from build123d import *

# Parameters (mm, degrees)
SKETCH1_W           = 10
SKETCH1_H           = 10
BOSS_EXTRUDE1_DEPTH = 8
SKETCH2_W           = 4
SKETCH2_H           = 3
CUT_EXTRUDE1_DEPTH  = 11
SKETCH3_W           = 1.504859188
SKETCH3_H           = 7
BOSS_EXTRUDE2_DEPTH = 3.5
FILLET1_R           = 2


with BuildPart() as part:
    # Sketch1 → Boss-Extrude1 (new body)
    with BuildSketch(Plane.XY):
        Rectangle(SKETCH1_W, SKETCH1_H)
    extrude(amount=BOSS_EXTRUDE1_DEPTH)

    # Sketch2 → Cut-Extrude1 (cut, through all)
    with BuildSketch(Plane.XZ.offset(5)):
        with Locations((0, 4)):
            Rectangle(SKETCH2_W, SKETCH2_H)
    extrude(amount=-CUT_EXTRUDE1_DEPTH, mode=Mode.SUBTRACT)

    # Sketch3 → Boss-Extrude2 (add)
    with BuildSketch(Plane.XY.offset(8)):
        Rectangle(SKETCH3_W, SKETCH3_H)
    extrude(amount=BOSS_EXTRUDE2_DEPTH)

    # Fillet1
    fillet1_edges = [part.edges().sort_by_distance(p)[0] for p in [
        (0, -5, 0),
        (-5, 0, 0),
        (0, 5, 0),
        (5, 0, 0),
        (5, -5, 4),
        (-5, -5, 4),
        (-5, 5, 4),
        (5, 5, 4),
    ]]
    fillet(fillet1_edges, radius=FILLET1_R)


solid = part.part
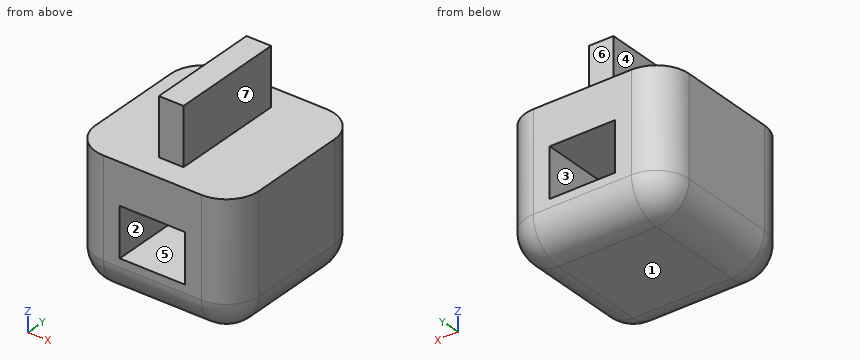
Can you work these out from the model? Positions are in its coordinate system, mm. Face numbers are marked on the shaded views. A direction names the side the tool comes from. Round coordinates to 2 decimals unless told otherwise and drop trailing zeros. Write each loop counter-clockwise with the first axis right and the second up, starting at its lowest first coordinate (ties: lowest second). Pieces come first, ordered by that corner, then holes. Notation, with made-up numbers: M 36,-34.5 L 57,-34.5 A8 cw 57,-22.5 Z; hole C 37,84.25 d4. An arc over 180 degrees is marked long. Use CSV: the item, a comma, the result in double quotes.
(1) We'd pull the mould along Z, two halves only. Please class the marked faces 1, 2, 3 and 4: +Z half, -Z half, draft (parallel to the pull), parting line (faces both ways), or undercut.
Check values:
face 1,"-Z half"
face 2,"undercut"
face 3,"undercut"
face 4,"draft"
(2) Imagine slicing it at A-A (y = 0.25). Write out the boundary of the cut face in (x, z), plus the area to 4 significant figures.
Check values:
outline,"M -5,2 A2 ccw -3,0 L 3,0 A2 ccw 5,2 L 5,8 L 0.75,8 L 0.75,11.5 L -0.75,11.5 L -0.75,8 L -5,8 Z; hole M -2,2.5 L 2,2.5 L 2,5.5 L -2,5.5 Z"
area,"71.55 mm^2"
(3) Imagine slicing it at B-B (x = -1). Write out the boundary of the cut face in (y, z).
Check values:
outline,"M -5,2 A2 ccw -3,0 L 3,0 A2 ccw 5,2 L 5,2.5 L -5,2.5 Z; M -5,5.5 L 5,5.5 L 5,8 L -5,8 Z"
(4) I'm going to push flat-ended pins straight in: pin 1 (1.7 mm diameter, centred on x = 0, z = 10.5, fed in from -Y); pin 2 (1 mm diameter, centred on y = 1, z = 9, fed in from -X); pin 3 (1.8 mm diameter, centred on y = 0.5, z = 10.5, fed in from +X). Where does each tip first touch, or does it pass through?
Check values:
pin 1,"y = -3.5"
pin 2,"x = -0.75"
pin 3,"x = 0.75"
(5) On a 3-axis mill with a long thin cutter (end or side, diameter ignored), from which of +Z, -Z, +X, -X, +Y, -Y can I reach the whole of each face in a straight line? I mean the marked faces 5, 6 and 7. Say none if no direction works.
Check values:
face 5,"+Y, -Y"
face 6,"+Z, +X, -X, +Y"
face 7,"+Z, +X, +Y, -Y"
(6) Imagine slicing it at D-D (y = -3.25). Write out the boundary of the cut face in (x, z).
Check values:
outline,"M -4.98,2 A1.98 ccw -3,0.02 L 3,0.02 A1.98 ccw 4.98,2 L 4.98,8 L 0.75,8 L 0.75,11.5 L -0.75,11.5 L -0.75,8 L -4.98,8 Z; hole M -2,2.5 L 2,2.5 L 2,5.5 L -2,5.5 Z"
(7) I need wall thicknesses on line 1 along X through (y, z) = (-0.5, 4.5); line 2 along X through (y, z) = (4.5, 4.5); line 3 along X through (y, z) = (2, 9.25). Which ranges of each line are inside material? Lowest first, please.
Check values:
line 1,"-5 to -2, 2 to 5"
line 2,"-4.32 to -2, 2 to 4.32"
line 3,"-0.75 to 0.75"
(8) Imagine slicing it at C-C (z = 7). Write out the boundary of the cut face in (x, y), plus the area to 3 significant figures.
Check values:
outline,"M -5,-3 A2 ccw -3,-5 L 3,-5 A2 ccw 5,-3 L 5,3 A2 ccw 3,5 L -3,5 A2 ccw -5,3 Z"
area,"96.6 mm^2"
